Input: part model. Units: mm. Frame: model coordinates. A direction names the side the tool comes from. Give positions to 0.01 mm unless a question says otherwise; leave off trailing zeros. Loops run counter-clockwise (first coordinate to the right, second up) from the corner with the lowest first, then second, coordinate; pieces in that order, holes last. Notation, with made-up numbers: (-28.75, 85) - (16.25, 85) arc R20 cw to (16.25, 113) - close; hole circle Ø2 at (87.5, 33.5). An arc over 180 degrees is marked (long way). One line per item, written item: value.
from build123d import *

# Parameters (mm, degrees)
SKETCH2_R                = 40
BOSS_EXTRUDE1_DEPTH      = 35
SKETCH3_W                = 8
SKETCH3_H                = 35
CUT_EXTRUDE1_DEPTH       = 20
SKETCH4_R                = 3.5
CUT_EXTRUDE2_DEPTH       = 80
SKETCH5_R                = 3.5
CUT_EXTRUDE3_DEPTH       = 50
SKETCH6_R                = 3.5
CUT_EXTRUDE4_DEPTH       = 50
SKETCH8_W                = 14.038446545
SKETCH8_H                = 6.5
CUT_EXTRUDE5_DEPTH       = 15.5
SKETCH11_W               = 8
SKETCH11_H               = 6.5
BOSS_EXTRUDE2_DEPTH      = 4.5
BOSS_EXTRUDE3_DEPTH      = 15.5
BOSS_EXTRUDE4_DEPTH      = 35
SKETCH18_R               = 3.5
CUT_EXTRUDE9_DEPTH       = 25
SKETCH19_R               = 3.5
CUT_EXTRUDE10_DEPTH      = 25
SKETCH20_R               = 3.5
CUT_EXTRUDE11_DEPTH      = 25
SKETCH21_W               = 5.1
SKETCH21_H               = 18.4
CUT_EXTRUDE12_DEPTH      = 13
SKETCH23_W               = 5.1
SKETCH23_H               = 18.4
CUT_EXTRUDE13_DEPTH      = 13
SKETCH22_W               = 5.1
SKETCH22_H               = 13.3
BOSS_EXTRUDE5_DEPTH      = 7.9
CUT_EXTRUDE14_DEPTH      = 8.5
SKETCH25_R               = 9
CUT_EXTRUDE15_DEPTH      = 20
SKETCH27_W               = 14.038446545
SKETCH27_H               = 6.5
CUT_EXTRUDE16_DEPTH      = 13
SKETCH28_R               = 3.5
CUT_EXTRUDE18_DEPTH      = 18
CUT_EXTRUDE18_DEPTH_BACK = 50


with BuildPart() as part:
    # Sketch2 → Boss-Extrude1 (new body)
    with BuildSketch(Plane.XY):
        Circle(SKETCH2_R)
    extrude(amount=BOSS_EXTRUDE1_DEPTH)

    # Sketch3 → Cut-Extrude1 (cut)
    with BuildSketch(Plane(origin=(0, 0, 0), x_dir=(-1, 0, 0), z_dir=(0, 0, -1))):
        with Locations((0, 21.5)):
            Rectangle(SKETCH3_W, SKETCH3_H)
        Polygon((31.774990748, -22.964101615), (35.774990748, -16.035898385), (5.464101615, 1.464101615), (1.464101615, -5.464101615), align=None)
        Polygon((-35.774990748, -16.035898385), (-31.774990748, -22.964101615), (-1.464101615, -5.464101615), (-5.464101615, 1.464101615), align=None)
    extrude(amount=-CUT_EXTRUDE1_DEPTH, mode=Mode.SUBTRACT)

    # Sketch4 → Cut-Extrude2 (cut)
    with BuildSketch(Plane(origin=(-3.464101615, -2, 0), x_dir=(0, 0, 1), z_dir=(-0.866025404, -0.5, 0))):
        with Locations((10, 0)):
            Circle(SKETCH4_R)
    extrude(amount=CUT_EXTRUDE2_DEPTH, mode=Mode.SUBTRACT)

    # Sketch5 → Cut-Extrude3 (cut)
    with BuildSketch(Plane(origin=(0, 4, 0), x_dir=(1, 0, 0), z_dir=(0, 1, 0))):
        with Locations((0, -10)):
            Circle(SKETCH5_R)
    extrude(amount=CUT_EXTRUDE3_DEPTH, mode=Mode.SUBTRACT)

    # Sketch6 → Cut-Extrude4 (cut)
    with BuildSketch(Plane(origin=(3.464101615, -2, 0), x_dir=(0, 0, -1), z_dir=(0.866025404, -0.5, 0))):
        with Locations((-10, 0)):
            Circle(SKETCH6_R)
    extrude(amount=CUT_EXTRUDE4_DEPTH, mode=Mode.SUBTRACT)

    # Sketch8 → Cut-Extrude5 (cut)
    with BuildSketch(Plane(origin=(0, 0, 0), x_dir=(-1, 0, 0), z_dir=(0, 0, -1))):
        Polygon((-32.971083956, -10.892407408), (-25.951860683, -23.050058746), (-20.322695558, -19.800058746), (-27.341918831, -7.642407408), align=None)
        with Locations((0.033217181, 30.75)):
            Rectangle(SKETCH8_W, SKETCH8_H)
        Polygon((27.30870165, -7.699941254), (32.937866774, -10.949941254), (25.918643502, -23.107592592), (20.289478377, -19.857592592), align=None)
    extrude(amount=-CUT_EXTRUDE5_DEPTH, mode=Mode.SUBTRACT)

    # Sketch11 → Boss-Extrude2 (add)
    with BuildSketch(Plane(origin=(0, 0, 20), x_dir=(-1, 0, 0), z_dir=(0, 0, -1))):
        with Locations((0, 30.75)):
            Rectangle(SKETCH11_W, SKETCH11_H)
        Polygon((25.815698604, -10.285898385), (31.444863729, -13.535898385), (27.444863729, -20.464101615), (21.815698604, -17.214101615), align=None)
        Polygon((-21.815698604, -17.214101615), (-27.444863729, -20.464101615), (-31.444863729, -13.535898385), (-25.815698604, -10.285898385), align=None)
    extrude(amount=BOSS_EXTRUDE2_DEPTH)

    # Sketch12 → Boss-Extrude3 (add)
    with BuildSketch(Plane(origin=(0, 0, 15.5), x_dir=(-1, 0, 0), z_dir=(0, 0, -1))):
        Polygon((-6.986006091, 32.1), (7.052440454, 32.1), (7.052440454, 34), (4, 34), (4, 39), (-4, 39), (-4, 34), (-6.986006091, 34), align=None)
        Polygon((25.918643502, -23.107592592), (27.444863729, -20.464101615), (31.774990748, -22.964101615), (35.774990748, -16.035898385), (31.444863729, -13.535898385), (32.937866774, -10.949941254), (31.292418507, -9.999941254), (24.273195235, -22.157592592), align=None)
        Polygon((-32.971083956, -10.892407408), (-31.444863729, -13.535898385), (-35.774990748, -16.035898385), (-31.774990748, -22.964101615), (-27.444863729, -20.464101615), (-25.951860683, -23.050058746), (-24.306412416, -22.100058746), (-31.325635688, -9.942407408), align=None)
    extrude(amount=BOSS_EXTRUDE3_DEPTH)

    # Sketch17 → Boss-Extrude4 (add)
    with BuildSketch(Plane(origin=(0, 0, 0), x_dir=(-1, 0, 0), z_dir=(0, 0, -1))):
        Polygon((-5.842787082, 32.897450406), (-5.842787082, 43.509531182), (5.727819383, 43.509531182), (5.754751517, 32.897450406), align=None)
        Polygon((31.411421312, -11.388723161), (25.612652013, -21.432486209), (34.816449619, -26.715202685), (40.601752851, -16.69476355), align=None)
        Polygon((-25.568634231, -21.508727245), (-31.36740353, -11.464964197), (-40.544269002, -16.794328497), (-34.75896577, -26.814767633), align=None)
    extrude(amount=-BOSS_EXTRUDE4_DEPTH)

    # Sketch18 → Cut-Extrude9 (cut, symmetric)
    with BuildSketch(Plane(origin=(-37.680359311, -21.754765591, 0), x_dir=(0, 0, 1), z_dir=(-0.866025404, -0.5, 0))):
        with Locations((10, 0)):
            Circle(SKETCH18_R)
    extrude(amount=CUT_EXTRUDE9_DEPTH, both=True, mode=Mode.SUBTRACT)

    # Sketch19 → Cut-Extrude10 (cut, symmetric)
    with BuildSketch(Plane(origin=(37.680359311, -21.754765591, 0), x_dir=(0, 0, -1), z_dir=(0.866025404, -0.5, 0))):
        with Locations((-10, 0)):
            Circle(SKETCH19_R)
    extrude(amount=CUT_EXTRUDE10_DEPTH, both=True, mode=Mode.SUBTRACT)

    # Sketch20 → Cut-Extrude11 (cut, symmetric)
    with BuildSketch(Plane(origin=(0, 43.509531182, 0), x_dir=(1, 0, 0), z_dir=(0, 1, 0))):
        with Locations((0, -10)):
            Circle(SKETCH20_R)
    extrude(amount=CUT_EXTRUDE11_DEPTH, both=True, mode=Mode.SUBTRACT)

    # Sketch21 → Cut-Extrude12 (cut)
    with BuildSketch(Plane(origin=(0, 0, 0), x_dir=(-1, 0, 0), z_dir=(0, 0, -1))):
        with Locations((6.55, 13.2)):
            Rectangle(SKETCH21_W, SKETCH21_H)
    extrude(amount=-CUT_EXTRUDE12_DEPTH, mode=Mode.SUBTRACT)

    # Sketch23 → Cut-Extrude13 (cut)
    with BuildSketch(Plane(origin=(0, 0, 0), x_dir=(-1, 0, 0), z_dir=(0, 0, -1))):
        with Locations((6.55, 13.2)):
            Rectangle(SKETCH23_W, SKETCH23_H)
        Polygon((-1.085898385, -9.880831174), (1.464101615, -5.464101615), (17.398969045, -14.664101615), (14.848969045, -19.080831174), align=None)
        Polygon((-8.014101615, 5.880831174), (-5.464101615, 1.464101615), (-21.398969045, -7.735898385), (-23.948969045, -3.319168826), align=None)
    extrude(amount=-CUT_EXTRUDE13_DEPTH, mode=Mode.SUBTRACT)

    # Sketch22 → Boss-Extrude5 (add)
    with BuildSketch(Plane(origin=(0, 0, 0), x_dir=(-1, 0, 0), z_dir=(0, 0, -1))):
        with Locations((6.55, 10.65)):
            Rectangle(SKETCH22_W, SKETCH22_H)
        Polygon((-1.085898385, -9.880831174), (1.464101615, -5.464101615), (12.982239485, -12.114101615), (10.432239485, -16.530831174), align=None)
        Polygon((-8.014101615, 5.880831174), (-5.464101615, 1.464101615), (-16.982239485, -5.185898385), (-19.532239485, -0.769168826), align=None)
    extrude(amount=-BOSS_EXTRUDE5_DEPTH)

    # Sketch24 → Cut-Extrude14 (cut)
    with BuildSketch(Plane.XY.offset(35)):
        with BuildLine():
            Line((0.831568399, -1), (1.11810064, -0.999925477))
            ThreePointArc((1.11810064, -0.999925477), (0.535186435, 1.401276375), (-1.5, 0))
            ThreePointArc((-1.5, 0), (-1.401274891, -0.535190321), (-1.118095094, -0.999931678))
            Line((-1.118095094, -0.999931678), (-0.831313787, -1))
            Line((-0.831313787, -1), (0.831568399, -1))
        make_face()
    extrude(amount=-CUT_EXTRUDE14_DEPTH, mode=Mode.SUBTRACT)

    # Sketch25 → Cut-Extrude15 (cut)
    with BuildSketch(Plane(origin=(0, 0, 0), x_dir=(-1, 0, 0), z_dir=(0, 0, -1))):
        Circle(SKETCH25_R)
    extrude(amount=-CUT_EXTRUDE15_DEPTH, mode=Mode.SUBTRACT)

    # Sketch27 → Cut-Extrude16 (cut)
    with BuildSketch(Plane.XY.offset(35)):
        with Locations((0.000904033, -14.25)):
            Rectangle(SKETCH27_W, SKETCH27_H)
    extrude(amount=-CUT_EXTRUDE16_DEPTH, mode=Mode.SUBTRACT)

    # Sketch28 → Cut-Extrude18 (cut, two sides)
    with BuildSketch(Plane(origin=(0, -17.5, 0), x_dir=(1, 0, 0), z_dir=(0, 1, 0))) as cut_extrude18_sk:
        with Locations((0, -27.44)):
            Circle(SKETCH28_R)
    extrude(amount=CUT_EXTRUDE18_DEPTH, mode=Mode.SUBTRACT)
    extrude(cut_extrude18_sk.sketch, amount=-CUT_EXTRUDE18_DEPTH_BACK, mode=Mode.SUBTRACT)


solid = part.part
Item 1: Material intervals for L1, parallel to Y at x = 0, z = 32.5; L2, parallel to X at y = -13, z = 4; L3, parallel to X at y = 37, z = 10, sorted ascending.
Verdict:
L1: y = -40 to -17.5, -11 to -1, 1.5 to 43.51
L2: x = -37.83 to -29.56, -12.47 to 14.52, 29.56 to 37.83
L3: x = -15.2 to -3.5, 3.5 to 15.2
Item 2: Pin query (flat end, axial travel): P1, Ø10, axis at x = -25, z = 25.5, coming from the +Y side; P2, Ø1, axis at y = 21.5, z = 7, coming from the +X side; P3, Ø9.5, axis at y = 17, z = 14.5, coming from the +X side. Return the tip coordinate at first contact, or that it passes through.
Verdict:
P1: stops at y = 34.64
P2: stops at x = 34.04
P3: stops at x = 38.08
Item 3: Section D-D, the plane y = -31.5. Output: boundary loops of the cut face in (x, z).
Verdict:
outline: (-24.65, 0) - (24.65, 0) - (24.65, 35) - (-24.65, 35) - close; hole circle Ø7 at (0, 27.44)
Item 4: Draft query along Z for faces 5 (the face through (-7, 12, 7.9)), 6 (the face through (0, 30, 15.5)), 7 (the face through (34.92, 19.51, 17.26)). Return one class per face: pulls with the +Z half, pulls with the -Z half, needs draft (parallel to the pull), parting line crosses it, or undercut.
Verdict:
face 5: undercut
face 6: pulls with the -Z half
face 7: needs draft
Item 5: Section A-A, the plane z = 18. Output: boundary loops of the cut face in (x, y).
Verdict:
outline: (-40.6, -16.69) - (-34.82, -26.72) - (-31.41, -24.76) arc R40 ccw to (31.35, -24.85) - (34.76, -26.81) - (40.54, -16.79) - (37.15, -14.82) arc R40 ccw to (5.84, 39.57) - (5.84, 43.51) - (-5.73, 43.51) - (-5.74, 39.59) arc R40 ccw to (-37.19, -14.73) - close; hole (-25.82, -10.29) - (-21.82, -17.21) - (-4.98, -7.5) arc R9 ccw to (4.98, -7.5) - (21.82, -17.21) - (25.82, -10.29) - (8.98, -0.57) arc R9 ccw to (4, 8.06) - (4, 27.5) - (-4, 27.5) - (-4, 8.06) arc R9 ccw to (-8.98, -0.57) - close
Item 6: Section B-B, the plane y = 33.5. Output: boundary loops of the cut face in (x, z).
Verdict:
outline: (-21.86, 0) - (21.86, 0) - (21.86, 35) - (-21.86, 35) - close; hole circle Ø7 at (0, 10)
Item 7: Section C-C, the plane z = 10. Count the separate pieces of the cut face and the enclosed holes in it, and give its area (3 significant figures).
Verdict:
separate pieces: 3
enclosed holes: 0
area: 3,760 mm^2
Item 8: Access query for faces 1 (the face through (-34.36, 20.48, 17.26)), 2 (the face through (4, 18, 10)), 3 (the face through (0, 0.5, 26)), 4 (the face through (-7.018, -14, 29)). Directions: +Z, -Z, +X, -X, +Y, -Y. A direction counts if a zero-diameter tool reaches every point of the face in a straight line with its end or side. Return the directions, or none.
Verdict:
face 1: +Z, -Z, -X
face 2: -Z
face 3: -Y
face 4: +Z
